Here's how the part is built. I have some questions about the finished solid (model axes, mm). A direction names the side the tool comes from. Give positions to 0.01 mm unless a question says otherwise; leave off trailing zeros. Write each loop counter-clockwise with the first axis right and the second up, starting at its lowest first coordinate (ties: lowest second). Pieces come first, ordered by that corner, then holes. Notation, with made-up numbers: (-12, 13.5) -> (33, 13.5) arc R24 ccw to (33, 43.5) -> close; hole circle Ø5 at (82.5, 56). An arc over 180 degrees is marked (long way). Answer as CSV lines item,"result". Start each with the question number.
from build123d import *

# Parameters (mm, degrees)
SKETCH1_W           = 44
SKETCH1_H           = 42
BOSS_EXTRUDE1_DEPTH = 56
BOSS_EXTRUDE2_DEPTH = 5
FILLET1_R           = 1


with BuildPart() as part:
    # Sketch1 → Boss-Extrude1 (new body)
    with BuildSketch(Plane.XY):
        with Locations((22, 21)):
            Rectangle(SKETCH1_W, SKETCH1_H)
    extrude(amount=-BOSS_EXTRUDE1_DEPTH)

    # Sketch2 → Boss-Extrude2 (add)
    with BuildSketch(Plane.XY):
        with BuildLine():
            Line((44, 42), (52.691651223, 42))
            ThreePointArc((52.691651223, 42), (47.065035319, 39.983558931), (44, 34.852243348))
            Line((44, 34.852243348), (44, 42))
        make_face()
    extrude(amount=-BOSS_EXTRUDE2_DEPTH)

    # Fillet1
    fillet1_edges = [part.edges().sort_by_distance(p)[0] for p in [
        (52.691651223, 42, -2.5),
    ]]
    fillet(fillet1_edges, radius=FILLET1_R)


solid = part.part
Item 1: If we section it at A-A (y = 21.5): Please give me the cut outline in (x, z).
Item 2: I'm going to push flat-ended pins straight in: pin 1 (2 mm diameter, centred on y = 22.5, z = -7.5, fed in from +X); pin 2 (1.1 mm diameter, centred on x = 46, y = 40, fed in from -Z). Where does each tip first touch, or does it pass through?
Item 3: If I drill on line 1 (X direction, y = 14.5, z = -18), over which ranges is the centre line in solid material (lowest first)? Write a range as [from, to].
Item 4: For faces 1 (the face through (22, 0, -28)), 2 (the face through (45, 40, -5)), which set-ups out of +Z, -Z, +X, -X, +Y, -Y let a thin tool reach every point of the face, with its end or its side?
Item 5: If we section it at B-B (x = 45.5): Please give me the cut outline in (y, z).
Final values:
1,outline,"(0, -56) -> (44, -56) -> (44, 0) -> (0, 0) -> close"
2,pin 1,"x = 44"
2,pin 2,"z = -5"
3,line 1,"[0, 44]"
4,face 1,"+Z, -Z, +X, -X, -Y"
4,face 2,"-Z, +X, +Y, -Y"
5,outline,"(38.31, -5) -> (42, -5) -> (42, 0) -> (38.31, 0) -> close"
